from build123d import *

# Parameters (mm, degrees)
F0_R     = 38.1
F0_R_2   = 25.4
F0_R_3   = 22.225
F1_DEPTH = 7.62
F2_DEPTH = 2.54
F3_D     = 6.7564


with BuildPart() as f1:
    # F0 (on Front) → F1 (new body)
    with BuildSketch(Plane.XZ):
        Circle(F0_R)
        with BuildLine():
            ThreePointArc((2.1860537536, 31.6746534154), (23.2106624925, 21.6639711655), (31.75, 0))
            ThreePointArc((31.75, 0), (30.9330089399, -7.15621813), (28.5240813906, -13.944148623))
            ThreePointArc((28.5240813906, -13.944148623), (29.3714883317, -14.7488554788), (29.6836584215, -15.875))
            ThreePointArc((29.6836584215, -15.875), (28.5571893518, -17.7878606445), (26.338027637, -17.7305047924))
            ThreePointArc((26.338027637, -17.7305047924), (0, -31.75), (-26.338027637, -17.7305047924))
            ThreePointArc((-26.338027637, -17.7305047924), (-29.3906088404, -16.9686759257), (-28.5240813906, -13.944148623))
            ThreePointArc((-28.5240813906, -13.944148623), (-27.4963065702, 15.875), (-2.1860537536, 31.6746534154))
            ThreePointArc((-2.1860537536, 31.6746534154), (-0.0376788829, 33.9370273028), (2.1873518513, 31.75))
            ThreePointArc((2.1873518513, 31.75), (2.1870273028, 31.7123211171), (2.1860537536, 31.6746534154))
        make_face(mode=Mode.SUBTRACT)
        with BuildLine():
            ThreePointArc((28.5240813906, -13.944148623), (30.9330089399, -7.15621813), (31.75, 0))
            ThreePointArc((31.75, 0), (23.2106624925, 21.6639711655), (2.1860537536, 31.6746534154))
            ThreePointArc((2.1860537536, 31.6746534154), (0, 29.5626481487), (-2.1860537536, 31.6746534154))
            ThreePointArc((-2.1860537536, 31.6746534154), (-27.4963065702, 15.875), (-28.5240813906, -13.944148623))
            ThreePointArc((-28.5240813906, -13.944148623), (-26.370162049, -13.9998182384), (-25.3089547188, -15.875))
            ThreePointArc((-25.3089547188, -15.875), (-25.5834459257, -16.9358827816), (-26.338027637, -17.7305047924))
            ThreePointArc((-26.338027637, -17.7305047924), (0, -31.75), (26.338027637, -17.7305047924))
            ThreePointArc((26.338027637, -17.7305047924), (25.6020042999, -14.7813240743), (28.5240813906, -13.944148623))
        make_face()
        Circle(F0_R_2, mode=Mode.SUBTRACT)
        Circle(F0_R_2)
        Circle(F0_R_3, mode=Mode.SUBTRACT)
        with BuildLine():
            ThreePointArc((-2.1860537536, 31.6746534154), (0, 31.75), (2.1860537536, 31.6746534154))
            ThreePointArc((2.1860537536, 31.6746534154), (2.1870273028, 31.7123211171), (2.1873518513, 31.75))
            ThreePointArc((2.1873518513, 31.75), (-0.0376788829, 33.9370273028), (-2.1860537536, 31.6746534154))
        make_face()
        with BuildLine():
            ThreePointArc((-2.1860537536, 31.6746534154), (0, 29.5626481487), (2.1860537536, 31.6746534154))
            ThreePointArc((2.1860537536, 31.6746534154), (0, 31.75), (-2.1860537536, 31.6746534154))
        make_face()
        with BuildLine():
            ThreePointArc((-26.338027637, -17.7305047924), (-27.4963065702, -15.875), (-28.5240813906, -13.944148623))
            ThreePointArc((-28.5240813906, -13.944148623), (-29.3906088404, -16.9686759257), (-26.338027637, -17.7305047924))
        make_face()
        with BuildLine():
            ThreePointArc((-25.3089547188, -15.875), (-26.370162049, -13.9998182384), (-28.5240813906, -13.944148623))
            ThreePointArc((-28.5240813906, -13.944148623), (-27.4963065702, -15.875), (-26.338027637, -17.7305047924))
            ThreePointArc((-26.338027637, -17.7305047924), (-25.5834459257, -16.9358827816), (-25.3089547188, -15.875))
        make_face()
        with BuildLine():
            ThreePointArc((29.6836584215, -15.875), (29.3714883317, -14.7488554788), (28.5240813906, -13.944148623))
            ThreePointArc((28.5240813906, -13.944148623), (27.4963065702, -15.875), (26.338027637, -17.7305047924))
            ThreePointArc((26.338027637, -17.7305047924), (28.5571893518, -17.7878606445), (29.6836584215, -15.875))
        make_face()
        with BuildLine():
            ThreePointArc((26.338027637, -17.7305047924), (27.4963065702, -15.875), (28.5240813906, -13.944148623))
            ThreePointArc((28.5240813906, -13.944148623), (25.6020042999, -14.7813240743), (26.338027637, -17.7305047924))
        make_face()
    extrude(amount=F1_DEPTH)

    # F0 (on Front) → F2 (cut)
    with BuildSketch(Plane.XZ):
        Circle(F0_R_2)
        Circle(F0_R_3, mode=Mode.SUBTRACT)
    extrude(amount=F2_DEPTH, mode=Mode.SUBTRACT)

    # F3 (through all)
    with Locations(Plane(origin=(0, 0, 0), x_dir=(1, 0, 0), z_dir=(0, 1, 0))):
        with Locations((27.4963065702, 15.875), (-27.4963065702, 15.875), (0, -31.75)):
            Hole(F3_D / 2)


solid = f1.part
Model file for the job. Use its own axes, mm. A direction names the side the tool comes from. Give positions to 0.01 mm unless a question says otherwise; leave off trailing zeros. Order: outer loops, then holes, each group sorted by start corner. A loop starts at its lowest first (then second) coordinate and runs counter-clockwise, first axis right, second up. Notation, with made-up numbers: (66, -14) - (104, -14) arc R13 cw to (104, 11) - close; hole circle Ø8 at (-38, 87.5). An arc over 180 degrees is marked (long way). One line per item, written item: value.
Item 1: Slice it at B-B (x = 0). List the corners of the cut face in (y, z) (3 decimals).
Response values:
outline: (-7.62, -38.1) - (0, -38.1) - (0, -25.4) - (-2.54, -25.4) - (-2.54, -22.225) - (-7.62, -22.225) - close; (-7.62, 22.225) - (-2.54, 22.225) - (-2.54, 25.4) - (0, 25.4) - (0, 28.372) - (-7.62, 28.372) - close; (-7.62, 35.128) - (0, 35.128) - (0, 38.1) - (-7.62, 38.1) - close
Item 2: Pin check, flat tips, straight feed: pin 1 Ø6 at (x, z) = (0, 31.75) entering from -Y (1 decimal); pin 2 Ø3 at (x, y) = (-21.5, -4) entering from +Z; pin 3 Ø4 at (y, z) = (-6, -27.5) entering from -X; pin 4 Ø3 at (y, z) = (-5.5, -12) entering from +X. Stop position of each tip, or through.
Response values:
pin 1: through
pin 2: z = 32.43
pin 3: x = -28.31
pin 4: x = 36.62
Item 3: Tool access for faces 4 (the flat face through (16, -7.62, -16)), 5 (the flat face through (-0.1, -2.54, -22.5)): list every direction of +Z, -Z, +X, -X, +Y, -Y with a clear straight run to the whole face (end or side of a thin tool).
Response values:
face 4: +Z, -Z, +X, -X, -Y
face 5: +Y
Item 4: Slice it at A-A (z = 0). List the corners of the cut face in (x, y) (3 decimals).
Response values:
outline: (-38.1, -7.62) - (-22.225, -7.62) - (-22.225, -2.54) - (-25.4, -2.54) - (-25.4, 0) - (-38.1, 0) - close; (22.225, -7.62) - (38.1, -7.62) - (38.1, 0) - (25.4, 0) - (25.4, -2.54) - (22.225, -2.54) - close
Item 5: Two-plate mould, pull along Z, no slides. Class faces 1 (the cylindrical face through (-30.235, -3.757, -23.183)), 2 (the cylindrical face through (-27.057, -3.863, -19.224)), 3 (the flat face through (8, 0, -25)): released by +Z, released by -Z, zero draft, split by the parting line, or undercut.
Response values:
face 1: split by the parting line
face 2: undercut
face 3: zero draft
Item 6: Slice it at D-D (y = -3.5). Give the number of separate pieces and of enclosed holes in the cut face, then the cut area to 3 significant figures.
Response values:
separate pieces: 1
enclosed holes: 4
area: 2,900 mm2
Item 7: Wall check: line 1 (Z direction, x = 0, y = -1.9); line 2 (X direction, y = -4.5, z = 0.5); line 3 (Y direction, x = 3.5, z = 23). Give the ranges that are in metal, low to high.
Response values:
line 1: -38.1 to -25.4, 25.4 to 28.37, 35.13 to 38.1
line 2: -38.1 to -22.22, 22.22 to 38.1
line 3: -7.62 to -2.54
Item 8: Slice it at C-C (x = 26.5). List the corners of the cut face in (y, z).
Response values:
outline: (-7.62, -27.37) - (0, -27.37) - (0, -19.1) - (-7.62, -19.1) - close; (-7.62, -12.65) - (0, -12.65) - (0, 27.37) - (-7.62, 27.37) - close
